Study the drawing (mm; zero at the part's minimum x, y, z) and answer. A direction names the side the tool comes from. Give positions to 0.01 mm unless a question says otherwise; leave off trailing zeros. Order: outer loops, then holes, each group sorted by start corner. A loop starts at its lowest first (then second) coordinate and runs counter-clockwise, first axis right, second up. Notation, with made-up numbers: (19.5, 52) - (31.5, 52) arc R26 ccw to (31.5, 72) - close; hole circle Ø7 at (57.5, 78). An arc over 180 degrees is marked (long way). Use CSV: the item, a comma, the result in double quotes.
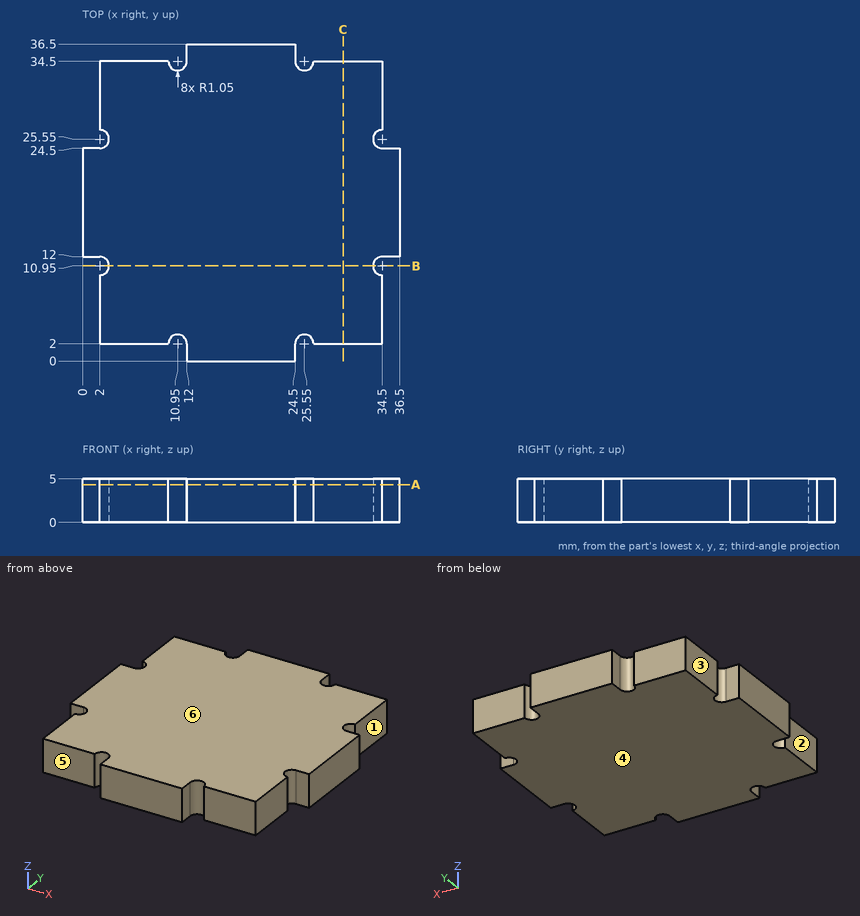
Item 1: The part is cut by section C-C (x = 30). Give the vertices of the cut face in (y, z), and give its area (4 significant figures).
Taken from the geometry:
outline,"(2, 0) - (34.5, 0) - (34.5, 5) - (2, 5) - close"
area,"162.5 mm^2"
Item 2: The part is cut by section B-B (y = 10.95). Give the vertices of the cut face in (x, z).
Taken from the geometry:
outline,"(3.05, 0) - (33.45, 0) - (33.45, 5) - (3.05, 5) - close"
Item 3: Each of these flat-tipped pins is pushed along its axis until it touches: pin 1 (1 mm diameter, centred on y = 36, z = 3, fed in from +X); pin 2 (1.5 mm diameter, centred on y = 7.5, z = 2.5, fed in from -X); pin 3 (1 mm diameter, centred on x = 35.5, z = 1.5, fed in from -Y). Where does it stop, or does it pass through?
Taken from the geometry:
pin 1,"x = 24.5"
pin 2,"x = 2"
pin 3,"y = 12"
Item 4: The part is cut by section A-A (z = 4.35). Give the vertices of the cut face in (x, y).
Taken from the geometry:
outline,"(0, 12) - (2, 12) arc R1.05 cw to (2, 9.9) - (2, 2) - (9.9, 2) arc R1.05 cw to (12, 2) - (12, 0) - (24.5, 0) - (24.5, 2) arc R1.05 cw to (26.6, 2) - (34.5, 2) - (34.5, 9.9) arc R1.05 cw to (34.5, 12) - (36.5, 12) - (36.5, 24.5) - (34.5, 24.5) arc R1.05 cw to (34.5, 26.6) - (34.5, 34.5) - (26.6, 34.5) arc R1.05 cw to (24.5, 34.5) - (24.5, 36.5) - (12, 36.5) - (12, 34.5) arc R1.05 cw to (9.9, 34.5) - (2, 34.5) - (2, 26.6) arc R1.05 cw to (2, 24.5) - (0, 24.5) - close"
Item 5: The mould has two halves that part along Z. Classify the marked faces 4, 5 and 6: +Z half, -Z half, draft (parallel to the pull), parting line (faces both ways), or undercut.
Taken from the geometry:
face 4,"-Z half"
face 5,"draft"
face 6,"+Z half"
Item 6: Which of the six approach directions +Z, -Z, +X, -X, +Y, -Y give full straight-line access (tool end or side, diameter ignored) to the marked faces 1, 2 and 3?
Taken from the geometry:
face 1,"+Z, -Z, +X, +Y"
face 2,"+Z, -Z, -X, -Y"
face 3,"+Z, -Z, -X, +Y"
Item 7: Find the intervals of material crossed by line 1 along Y through (x, z) = (34, 4.1); line 2 along X through (y, z) = (9, 0.9), in increasing order.
Taken from the geometry:
line 1,"2 to 10.03, 11.87 to 24.63, 26.47 to 34.5"
line 2,"2 to 34.5"
